Part model, mm, in its own coordinate system. Face numbers are marked on the shaded views. Round coordinates to 2 decimals unless told otherwise and drop trailing zeros. Write each loop counter-clockwise with the first axis right and the second up, starting at its lowest first coordinate (ties: lowest second). Pieces come first, ordered by that corner, then holes. Notation, with made-up numbers: M 65,25 L 97,25 A16 cw 97,42 Z; hole C -19,47 d3. An arc over 180 degrees is marked long. One line per question, with ' | ' between items. Start each with the question number.
1) Saw through at B-B (y = -42). List the corners of the cut face in (x, z), plus the area to 3 significant figures.
2) Mould opens along Z. For the marked faces 1, 2, 3 and 4 say: pulls with the +Z half, pulls with the -Z half, needs draft (parallel to the pull), parting line crosses it, or undercut.
3) Saw through at C-C (z = 0). List the corners of the cut face in (x, y).
4) Wall check: probe 1 along X at (y, z) = (-53.5, 0); probe 2 along Z at (x, y) = (-0.25, -48); probe 3 along X at (y, z) = (-49.5, -2.75). Give the ranges that are in metal, low to high. Write a range as [from, to].
5) Saw through at D-D (z = 6.25). List the corners of the cut face in (x, y).
6) Drop flat-ended pins along their axis: pin 1 Ø1 at (x, y) = (-3.5, -22.5) entering from -Z; pin 2 Ø5 at (y, z) = (-39, 2) entering from +X; pin 3 Ø6 at (x, y) = (5, 4.5) entering from -Z. Give the stop position or say it passes through.
7) Saw through at A-A (y = 48.5). List the corners of the cut face in (x, z).
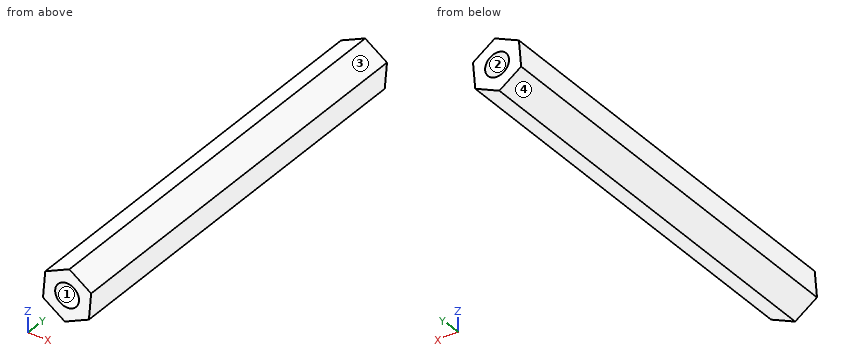
```python
from build123d import *

# Parameters (mm, degrees)
BOSS_EXTRUDE1_DEPTH = 57.15
SKETCH2_R           = 3.2893
CUT_EXTRUDE1_DEPTH  = 12.7


with BuildPart() as part:
    # Sketch1 → Boss-Extrude1 (new body, symmetric)
    with BuildSketch(Plane(origin=(0, 0, 0), x_dir=(1, 0, 0), z_dir=(0, 1, 0))):
        Polygon((6.016541477, 4.191009662), (-0.621250096, 7.305982593), (-6.637791573, 3.114972932), (-6.016541477, -4.191009662), (0.621250096, -7.305982593), (6.637791573, -3.114972932), align=None)
    extrude(amount=BOSS_EXTRUDE1_DEPTH, both=True)

    # Sketch2 → Cut-Extrude1 (cut)
    with BuildSketch(Plane(origin=(0, 57.15, 0), x_dir=(1, 0, 0), z_dir=(0, 1, 0))):
        Circle(SKETCH2_R)
    cut_extrude1 = extrude(amount=-CUT_EXTRUDE1_DEPTH, mode=Mode.SUBTRACT)

    # Mirror1: Cut-Extrude1 across plane
    add(cut_extrude1.mirror(Plane.ZX), mode=Mode.SUBTRACT)


solid = part.part
```
Answer key:
1) outline: M -6.64,-3.11 L -0.62,-7.31 L 6.02,-4.19 L 6.64,3.11 L 0.62,7.31 L -6.02,4.19 Z | area: 140 mm2
2) face 1: undercut | face 2: undercut | face 3: pulls with the +Z half | face 4: pulls with the -Z half
3) outline: M -6.37,-57.15 L -3.29,-57.15 L -3.29,-44.45 L 3.29,-44.45 L 3.29,-57.15 L 6.37,-57.15 L 6.37,57.15 L 3.29,57.15 L 3.29,44.45 L -3.29,44.45 L -3.29,57.15 L -6.37,57.15 Z
4) probe 1: x = [-6.37, -3.29], [3.29, 6.37] | probe 2: z = [-7.13, -3.28], [3.28, 6.9] | probe 3: x = [-6.61, -1.8], [1.8, 6.14]
5) outline: M -1.63,-57.15 L 2.14,-57.15 L 2.14,57.15 L -1.63,57.15 Z
6) pin 1: stops at z = -5.65 | pin 2: stops at x = 6.64 | pin 3: stops at z = -6.08
7) outline: M -6.64,-3.11 L -0.62,-7.31 L 6.02,-4.19 L 6.64,3.11 L 0.62,7.31 L -6.02,4.19 Z; hole C 0,0 d6.58
